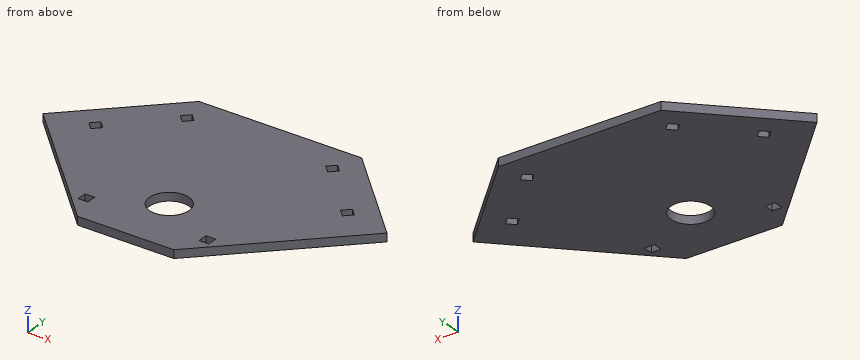
```python
from build123d import *

# Parameters (mm, degrees)
SKETCH3_R           = 12
BOSS_EXTRUDE1_DEPTH = 5
BOSS_EXTRUDE2_DEPTH = 5
SKETCH6_W           = 6
SKETCH6_H           = 6
CUT_EXTRUDE1_DEPTH  = 5


with BuildPart() as part:
    # Sketch3 → Boss-Extrude1 (new body)
    with BuildSketch(Plane.XY):
        Polygon((-77.781745931, 49.497474683), (-49.497474683, 77.781745931), (-43.840620434, 83.43860018), (43.840620434, 83.43860018), (49.497474683, 77.781745931), (77.781745931, 49.497474683), (88.388347648, 38.890872965), (27.497474683, -22), (-27.497474683, -22), (-88.388347648, 38.890872965), align=None)
        Circle(SKETCH3_R, mode=Mode.SUBTRACT)
        Polygon((-81.317279836, 44.547727215), (-77.074639149, 48.790367902), (-72.831998462, 44.547727215), (-77.074639149, 40.305086528), align=None, mode=Mode.SUBTRACT)
        Polygon((-48.790367902, 77.074639149), (-44.547727215, 81.317279836), (-40.305086528, 77.074639149), (-44.547727215, 72.831998462), align=None, mode=Mode.SUBTRACT)
        Polygon((40.305086528, 77.074639149), (44.547727215, 72.831998462), (48.790367902, 77.074639149), (44.547727215, 81.317279836), align=None, mode=Mode.SUBTRACT)
        Polygon((72.831998462, 44.547727215), (77.074639149, 40.305086528), (81.317279836, 44.547727215), (77.074639149, 48.790367902), align=None, mode=Mode.SUBTRACT)
    extrude(amount=BOSS_EXTRUDE1_DEPTH)

    # Sketch5 → Boss-Extrude2 (add)
    with BuildSketch(Plane.XY.offset(5)):
        Polygon((-105.358910397, 38.890872965), (-49.811183182, 94.43860018), (49.811183182, 94.43860018), (105.358910397, 38.890872965), (29.468037432, -37), (-29.468037432, -37), align=None)
        Polygon((-43.840620434, 83.43860018), (-88.388347648, 38.890872965), (-27.497474683, -22), (27.497474683, -22), (88.388347648, 38.890872965), (43.840620434, 83.43860018), align=None, mode=Mode.SUBTRACT)
    extrude(amount=-BOSS_EXTRUDE2_DEPTH)

    # Sketch6 → Cut-Extrude1 (cut)
    with BuildSketch(Plane.XY.offset(5)):
        with Locations((-37, -19)):
            Rectangle(SKETCH6_W, SKETCH6_H)
        with Locations((37, -19)):
            Rectangle(SKETCH6_W, SKETCH6_H)
    extrude(amount=-CUT_EXTRUDE1_DEPTH, mode=Mode.SUBTRACT)


solid = part.part
```
Build history of the part. All positions in model axes, mm. Round coordinates to 2 decimals unless told otherwise and drop trailing zeros. Write each loop counter-clockwise with the first axis right and the second up, starting at its lowest first coordinate (ties: lowest second). Pieces come first, ordered by that corner, then holes. Notation, with made-up numbers: (62.5, 82.25) - (106.5, 82.25) arc R15 ccw to (106.5, 88.25) - close; hole circle Ø1 at (-19.5, -27.75). An arc over 180 degrees is marked (long way). Answer as CSV lines item,"result".
Q1. Drop flat-ended pins along their axis: pin 1 (2.5 mm diameter, centred on x = 36, z = 3, fed in from -Y); pin 2 (1.5 mm diameter, centred on x = -38.5, z = 2, fed in from -Y). Give the stop position or say it passes through.
Report:
pin 1,"stops at y = -31.72"
pin 2,"stops at y = -28.72"
Q2. Cut at D-D (y = 61.5). Write the cut outline in (x, z), and give its area (4 significant figures).
Report:
outline,"(-82.75, 0) - (82.75, 0) - (82.75, 5) - (-82.75, 5) - close"
area,"827.5 mm^2"
Q3. Drill centre lines: probe 1 along Y at (x, z) = (0, 3.4); probe 2 along X at (y, z) = (7, 3.6); probe 3 along Y at (x, z) = (41, 3.1). Where is each one in solid material? Low to high. Write a range as [from, to].
Report:
probe 1,"y = [-37, -12], [12, 94.44]"
probe 2,"x = [-73.47, -9.75], [9.75, 73.47]"
probe 3,"y = [-25.47, 76.38], [77.77, 94.44]"
Q4. Cut at B-B (x = 0). Write the cut outline in (y, z).
Report:
outline,"(-37, 0) - (-12, 0) - (-12, 5) - (-37, 5) - close; (12, 0) - (94.44, 0) - (94.44, 5) - (12, 5) - close"
Q5. Cut at C-C (y = 7). Write the cut outline in (x, z).
Report:
outline,"(-73.47, 0) - (-9.75, 0) - (-9.75, 5) - (-73.47, 5) - close; (9.75, 0) - (73.47, 0) - (73.47, 5) - (9.75, 5) - close"
Q6. Cut at A-A (z = 4.25). State how many separate pieces and enclosed holes the cut face has, and give its area (3 significant figures).
Report:
separate pieces,"1"
enclosed holes,"7"
area,"18,200 mm^2"
